Verification items for the finished model (mm, model axes). Face numbers are marked on the shaded views. A direction names the side the tool comes from. Round coordinates to 2 decimals unless told otherwise and drop trailing zeros. Order: outer loops, then holes, each group sorted by start corner. A loop starts at its lowest first (then second) coordinate and runs counter-clockwise, first axis right, second up. Notation, with made-up numbers: (21, -23.75) -> (44, -23.75) arc R20 ccw to (44, -16.75) -> close; hole circle Ø10 at (76, -20.75). An arc over 180 degrees is marked (long way). Write item = value, one per line. Start each with the question number.
from build123d import *

# Parameters (mm, degrees)
SKETCH1_R               = 4.7625
BOSS_EXTRUDE1_DEPTH     = 66.675
SKETCH1_4_R             = 9.525
SKETCH1_4_R_2           = 0.800000051
SKETCH1_4_R_3           = 4.7625
SKETCH1_4_R_4           = 3.175
BOSS_EXTRUDE2_DEPTH     = 4.7625
FILLET1_R               = 3.175
SKETCH3_R               = 1.399999994
CUT_EXTRUDE2_DEPTH      = 10.525
CUT_EXTRUDE2_DEPTH_BACK = 10.525
SKETCH4_R               = 1.399999994
CUT_EXTRUDE3_DEPTH      = 12.03429274
CUT_EXTRUDE3_DEPTH_BACK = 12.03429274
SKETCH5_R               = 1.399999994
CUT_EXTRUDE4_DEPTH      = 12.03429274
CUT_EXTRUDE4_DEPTH_BACK = 12.03429274


with BuildPart() as part:
    # Sketch1 → Boss-Extrude1 (new body)
    with BuildSketch(Plane.XY):
        Circle(SKETCH1_R)
    extrude(amount=BOSS_EXTRUDE1_DEPTH)

    # Sketch1<4> → Boss-Extrude2 (add)
    with BuildSketch(Plane.XY):
        Circle(SKETCH1_4_R)
        with Locations((-6.99999997, 0)):
            Circle(SKETCH1_4_R_2, mode=Mode.SUBTRACT)
        with Locations((0, -6.99999997)):
            Circle(SKETCH1_4_R_2, mode=Mode.SUBTRACT)
        with Locations((6.99999997, 0)):
            Circle(SKETCH1_4_R_2, mode=Mode.SUBTRACT)
        with Locations((0, 6.99999997)):
            Circle(SKETCH1_4_R_2, mode=Mode.SUBTRACT)
        Circle(SKETCH1_4_R_3, mode=Mode.SUBTRACT)
        Circle(SKETCH1_4_R_3)
        Circle(SKETCH1_4_R_4, mode=Mode.SUBTRACT)
    extrude(amount=-BOSS_EXTRUDE2_DEPTH)

    # Fillet1
    fillet1_edges = [part.edges().sort_by_distance(p)[0] for p in [
        (-3.175, 0, 0),
    ]]
    fillet(fillet1_edges, radius=FILLET1_R)

    # Sketch3 → Cut-Extrude2 (cut, two sides)
    with BuildSketch(Plane(origin=(0, 0, 0), x_dir=(0, 0, -1), z_dir=(1, 0, 0))) as cut_extrude2_sk:
        with Locations((-38.89375, 0)):
            Circle(SKETCH3_R)
    extrude(amount=CUT_EXTRUDE2_DEPTH, mode=Mode.SUBTRACT)
    extrude(cut_extrude2_sk.sketch, amount=-CUT_EXTRUDE2_DEPTH_BACK, mode=Mode.SUBTRACT)

    # Sketch4 → Cut-Extrude3 (cut, two sides)
    with BuildSketch(Plane(origin=(0, 0, 0), x_dir=(0, 0, -1), z_dir=(0.173648178, 0.984807753, 0))) as cut_extrude3_sk:
        with Locations((-53.18125, 0)):
            Circle(SKETCH4_R)
    extrude(amount=CUT_EXTRUDE3_DEPTH, mode=Mode.SUBTRACT)
    extrude(cut_extrude3_sk.sketch, amount=-CUT_EXTRUDE3_DEPTH_BACK, mode=Mode.SUBTRACT)

    # Sketch5 → Cut-Extrude4 (cut, two sides)
    with BuildSketch(Plane(origin=(0, 0, 0), x_dir=(0, 0, -1), z_dir=(-0.173648178, 0.984807753, 0))) as cut_extrude4_sk:
        with Locations((-24.60625, 0)):
            Circle(SKETCH5_R)
    extrude(amount=CUT_EXTRUDE4_DEPTH, mode=Mode.SUBTRACT)
    extrude(cut_extrude4_sk.sketch, amount=-CUT_EXTRUDE4_DEPTH_BACK, mode=Mode.SUBTRACT)


solid = part.part
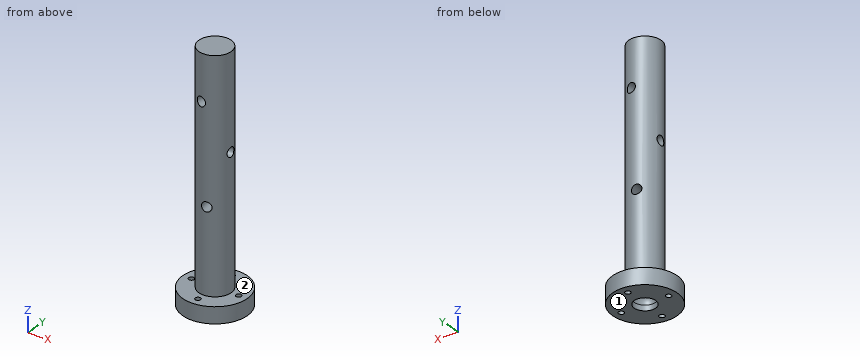
(1) Scan lines: line 1 along Y through (x, z) = (0, -2.8) (3 decimals); line 2 along Y through (x, z) = (0, -2.3) (3 decimals); line 3 along Z through (x, y) = (3.5, 0) (1 decimal). Record each from-to range of solid material in increasing order. Write a range as from..to.
(2) Cross-section at C-C (z = 39). Enter the section's corners in (x, y) (1 decimal), and give its area (3 significant figures).
(3) Cross-section at A-A (y = -7). Enter the section's corners in (x, z), and give its area (3 significant figures).
(4) Set-up check for the marked faces 1 and 2: record each of +Z, -Z, +X, -X, +Y, -Y from which the full face is reachable in a straight line by a thin tool's end or side.
(5) Cross-section at D-D (z = 10.5). Enter the section's corners in (x, y) (1 decimal).
(6) Depth check by flat-ended pin: pin 1 (10 mm diameter, centred on x = 4.5, z = 27, fed in from -Y); pin 2 (1.5 mm diameter, centred on x = 5, z = 4, fed in from -Y); pin 3 (1.8 mm diameter, centred on x = 0, y = 7, fed in from +Z); pin 4 (1 mm diameter, centred on x = -7, y = 0, fed in from -Z). Enter the tip coordinate at first touch or a pass-through.
Outcome:
q1.line_1 = -9.525..-7.8, -6.2..-3.153, 3.153..6.2, 7.8..9.525
q1.line_2 = -9.525..-7.8, -6.2..-3.052, 3.052..6.2, 7.8..9.525
q1.line_3 = -4.8..37.5, 40.3..66.7
q2.outline = (-4.6, -1.4) arc R4.8 ccw to (4.6, -1.4) -> close; (-4.6, 1.4) -> (4.6, 1.4) arc R4.8 ccw to start
q2.area = 45.0 mm^2
q3.outline = (-6.46, -4.76) -> (-0.8, -4.76) -> (-0.8, 0) -> (-6.46, 0) -> close; (0.8, -4.76) -> (6.46, -4.76) -> (6.46, 0) -> (0.8, 0) -> close
q3.area = 53.9 mm^2
q4.face_1 = -Z, +X, -X, +Y, -Y
q4.face_2 = +Z
q5.outline = circle Ø9.5 at (0, 0)
q6.pin_1 = -4.76
q6.pin_2 = -2.15
q6.pin_3 = 0
q6.pin_4 = through
